CAD build for the part. Positions are in the model's coordinates, mm. A direction names the side the tool comes from. Coordinates: 2 decimals unless noted, no trailing zeros. Order: outer loops, then holes, each group sorted by start corner. A loop starts at its lowest first (then second) coordinate and runs counter-clockwise, first axis right, second up. Notation, with made-up numbers: (43.5, 12) - (94.5, 12) arc R14 ccw to (94.5, 29) - close; hole circle Ø4 at (27, 10.5). An arc over 180 degrees is marked (long way). Write each question's results on one line, items separated by ' | '. Start each with the question number.
Q1. Band-saw the part on B-B, the plane y = -12.5. Write the cut outline in (x, z).
Q2. Band-saw the part on C-C, the plane z = 32. Write the cut outline in (x, y).
Q3. Band-saw the part on A-A, the plane x = -17. Write the cut outline in (y, z).
Q4. Pin check, flat tips, straight feed: P1, Ø1.2, axis at x = -26, z = 1, coming from the +Y side; P2, Ø5, axis at x = -9.51, y = -7.5, coming from the +Z side; P3, Ø10.5, axis at y = 8.5, z = 14.5, coming from the -X side. Stop position of each tip, or through.
Q5. Pull direction Y, two halves, no side cores. Call faces 1 (the cylindrical face through (0.76, 19.43, 37.9)), 2 (the flat face through (0, 0, 21)), 3 (the cylindrical face through (-36.97, 6.89, 0.74)): released by +Y, released by -Y, zero draft, split by the parting line, or undercut.
Q6. Wall check: probe 1 along Y at (x, z) = (-22.5, 0.8); probe 2 along Z at (x, y) = (0.3, 16.55); probe 3 along X at (y, z) = (-7, 1) (3 decimals). Give the ranges that are in metal, low to high.
Q7. Which spindle directions (+Z, -Z, +X, -X, +Y, -Y) get a long thin tool onto all of the face, cutting with end or side? Do faces 4 (the flat face through (-23, 6.5, 1)), 5 (the flat face through (-18, -9, 0)), 6 (the flat face through (-18, -9, 1.5)). Say none if no direction does.
Q8. Band-saw the part on D-D, the plane y = -5. Write the cut outline in (x, z), then the cut area to 3 significant figures.
Autodesk Inventor part; units mm, degrees
ref_plane "YZ Plane" through (0, 0, 0) normal (1, 0, 0) x (0, 1, 0)
ref_plane "XZ Plane" through (0, 0, 0) normal (0, 1, 0) x (-1, 0, 0)
ref_plane "XY Plane" through (0, 0, 0) normal (0, 0, 1) x (1, 0, 0)
sketch "Schizzo1" plane through (0, 0, 0) normal (0, 0, 1) x (1, 0, 0)
  line L0 (0, -20) -> (-22.5, -20)
  line L1 (-42.5, -20) -> (-42.5, 0)
  line L2 (-22.5, 20) -> (0, 20)
  line L3 (42.5, -20) -> (-42.5, 20) construction
  line L4 (-42.5, -20) -> (42.5, 20) construction
  arc A0 (-22.5, 20) -> (-22.5, -20) centre (-22.5, 0) ccw
  arc A1 (-2.5356, -1.1932) -> (-2.5356, 1.1932) centre (-22.5, 0) ccw
  line L5 (0, 20) -> (0, -20)
  point P0 (0, 0)
  dimension "d1" = 40
  dimension "d2" = 20
extrude "Piano1" add sketch "Schizzo1" along normal blind 1.5
sketch "Schizzo2" plane through (0, 0, 1.5) normal (0, 0, 1) x (1, 0, 0)
  line L0 (-22.5, 20) -> (0, 20)
  point P0 (0, 0)
sketch "Schizzo3" plane through (0, 20, 1.5) normal (1, 0, 0) x (0, 1, 0)
  line L0 (-40, 0) -> (0, 0)
  line L1 (0, 0) -> (0, 37)
  line L2 (0, 37) -> (-40, 37)
  line L3 (-40, 37) -> (-40, 0)
edge flange "Flangia1" height 38.5 angle 90 thickness 1.5 bend radius 1.5 thickness toward (1, 0, 0) relief tear relief width 1.5 relief depth 0.75 edges at (0, 0, 1.5) wall of the first edge with corners at (0, -20, 1.5) (0, 20, 1.5) (0, 20, 38.5) (0, -20, 38.5)
bend "Piega (Bend)1"
corner "Angolo1"
sketch "Schizzo4" plane through (1.5, -20, 38.5) normal (1, 0, 0) x (0, 0, -1)
  circle A0 centre (6.5, 36.55) radius 1.75
  line L0 (0, 0) -> (0, 40)
  line L1 (0, 40) -> (35.5, 40)
  circle A1 centre (29.75, 36.55) radius 1.75
  circle A2 centre (6.5, 6.55) radius 1.75
  circle A3 centre (29.75, 6.55) radius 1.75
  point P0 (38.5, 20)
  dimension "d15" = 3.5
  dimension "d16" = 6.5
  dimension "d17" = 3.45
  dimension "d18" = 3.5
  dimension "d19" = 23.25
  dimension "d20" = 3.5
  dimension "d21" = 30
  dimension "d22" = 3.5
hole "Foro1" at (1.5, 16.55, 32) at (1.5, 16.55, 8.75) at (1.5, -13.45, 8.75) at (1.5, -13.45, 32) direction (-1, 0, 0) diameter 3.5 depth 1.5 tip angle 118
sketch "Schizzo5" plane through (0, 0, 0) normal (0, 0, -1) x (-1, 0, 0)
  line L0 (16.15, 0) -> (29.4, 0) construction
  line L1 (16.15, -6.5) -> (29.4, -6.5)
  line L2 (29.4, 6.5) -> (16.15, 6.5)
  arc A0 (16.15, 6.5) -> (16.15, -6.5) centre (16.15, 0) ccw
  arc A1 (29.4, -6.5) -> (29.4, 6.5) centre (29.4, 0) ccw
  arc A2 (22.5, -20) -> (22.5, 20) centre (22.5, 0) ccw
  circle A3 centre (22.5, -15) radius 1.6
  circle A4 centre (35.4904, -7.5) radius 1.6
  circle A5 centre (35.4904, 7.5) radius 1.6
  circle A6 centre (22.5, 15) radius 1.6
  circle A7 centre (9.5096, 7.5) radius 1.6
  circle A8 centre (9.5096, -7.5) radius 1.6
  point P0 (0, 0)
  point P1 (22.775, 0)
  point P2 (42.5, 0)
  point P3 (35.9, 0)
  dimension "d30" = 13.25
  dimension "d31" = 13
  dimension "d32" = 6.6
  dimension "d33" = 3.2
  dimension "d34" = 15
  dimension "d39" = 360
extrude "Taglia1" cut sketch "Schizzo5" against normal blind 1.5
fillet "Arrotondamento angolo1" radius 2 2 edges at (0.75, 20, 38.5) (0.75, -20, 38.5)
equation "\"d28\" = Spessore"
equation "\"d41\" = Spessore"
equation "\"d3\" = Spessore"
equation "\"d5\" = LarghezzaScaricoPiega"
equation "\"d6\" = ProfonditàScaricoPiega"
equation "\"d7\" = ResiduoMinimo"
equation "\"d8\" = RaggioTransizione"
equation "\"d11\" = RaggioPiega"
equation "\"d12\" = DimensioniScaricoAngolo"
equation "\"d13\" = DimensioneGioco"
equation "\"d14\" = Dimensione_raggio_Jacobi"
equation "\"RaggioPiega\" = Spessore"
equation "\"LarghezzaScaricoPiega\" = Spessore"
equation "\"ProfonditàScaricoPiega\" = 0.5 * Spessore"
equation "\"DimensioniScaricoAngolo\" = 4 * Spessore"
equation "\"ResiduoMinimo\" = 2 * Spessore"
equation "\"RaggioTransizione\" = RaggioPiega"
equation "\"Dimensione_raggio_Jacobi\" = RaggioPiega"
equation "\"DimensioneGioco\" = Spessore"
properties part number "staffa motore"
Results below:
1) outline: (-38.11, 0) - (-1.5, 0) arc R3 ccw to (1.5, 3) - (1.5, 7.28) - (0, 7.28) - (0, 3) arc R1.5 cw to (-1.5, 1.5) - (-38.11, 1.5) - close; (0, 10.22) - (1.5, 10.22) - (1.5, 30.53) - (0, 30.53) - close; (0, 33.47) - (1.5, 33.47) - (1.5, 38.5) - (0, 38.5) - close
2) outline: (0, -20) - (1.5, -20) - (1.5, -15.2) - (0, -15.2) - close; (0, -11.7) - (1.5, -11.7) - (1.5, 14.8) - (0, 14.8) - close; (0, 18.3) - (1.5, 18.3) - (1.5, 20) - (0, 20) - close
3) outline: (-20, 0) - (-6.5, 0) - (-6.5, 1.5) - (-20, 1.5) - close; (6.5, 0) - (20, 0) - (20, 1.5) - (6.5, 1.5) - close
4) P1: stops at y = 19.79 | P2: stops at z = 1.5 | P3: stops at x = 0
5) face 1: released by +Y | face 2: zero draft | face 3: undercut
6) probe 1: y = -20 to -16.6, -13.4 to -6.5, 6.5 to 13.4, 16.6 to 20 | probe 2: z = 0.6 to 7, 10.5 to 30.25, 33.75 to 38.5 | probe 3: x = -41.235 to -37.01, -33.971 to -11.029, -7.99 to 0.736
7) face 4: +Z, -Z | face 5: -Z, +X, -X, +Y, -Y | face 6: +Z, -X, +Y, -Y
8) outline: (-41.86, 0) - (-33.55, 0) - (-33.55, 1.5) - (-41.86, 1.5) - close; (-12, 0) - (-1.5, 0) arc R3 ccw to (1.5, 3) - (1.5, 38.5) - (0, 38.5) - (0, 3) arc R1.5 cw to (-1.5, 1.5) - (-12, 1.5) - close | area: 86.8 mm²
